For this review, take the finished solid that the model builds, in its own axes (mm). Coordinates: 2 decimals unless noted, no trailing zeros. Write each loop counter-clockwise with the first axis right and the second up, starting at its lowest first coordinate (ties: lowest second). Pieces come first, ordered by that corner, then holes. Notation, with made-up numbers: M -22.5,-39 L 16.5,-39 A33 cw 16.5,-2 Z; hole C -7,-16.75 d3. An arc over 180 degrees is marked long. Return JSON: item names as keys, results as strings.
```python
from build123d import *

# Parameters (mm, degrees)
CYLINDER_R        = 15.5
CYLINDER_DEPTH    = 10
CYLINDER001_R     = 32.5
CYLINDER001_DEPTH = 1


with BuildPart() as cylinder:
    # Cylinder → Cylinder (new body)
    with BuildSketch(Plane.XY.offset(-2)):
        Circle(CYLINDER_R)
    extrude(amount=CYLINDER_DEPTH)


with BuildPart() as cut:
    # Cylinder001 → Cylinder001 (new body)
    with BuildSketch(Plane.XY):
        Circle(CYLINDER001_R)
    extrude(amount=CYLINDER001_DEPTH)

    # Cut: cut Cylinder
    add(cylinder.part, mode=Mode.SUBTRACT)


solid = cut.part
```
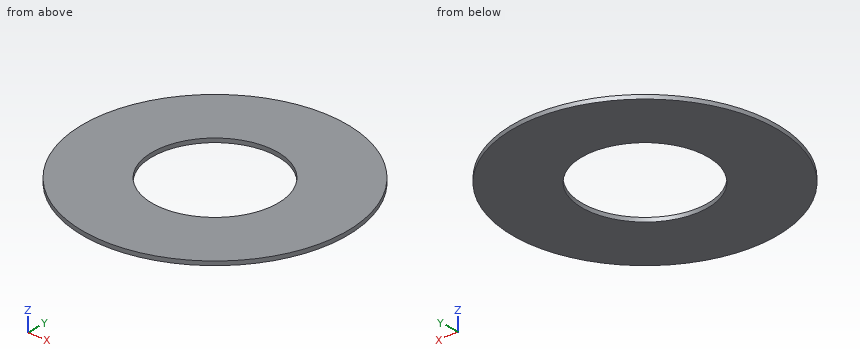
1. We need section D-D (x = -24.5). State the section outline as (y, z) points, plus the area to 3 significant figures.
Checks:
{"outline": "M -21.35,0 L 21.35,0 L 21.35,1 L -21.35,1 Z", "area": "42.7 mm2"}
2. We need section C-C (z = 0.7). State the section outline as (x, y) points, plus the area to 3 significant figures.
Checks:
{"outline": "C 0,0 d65; hole C 0,0 d31", "area": "2,560 mm2"}
3. Wall thickness on L1, parallel to Y at x = 0, z = 0.35; L2, parallel to Y at x = 2.5, z = 0.65; L3, parallel to Y at x = 21.5, z = 0.4: over which ranges is each line inside the solid? List them lowest first. Write a range as from..to.
Checks:
{"L1": "-32.5..-15.5, 15.5..32.5", "L2": "-32.4..-15.3, 15.3..32.4", "L3": "-24.37..24.37"}
4. We need section A-A (x = 0). State the section outline as (y, z) points, plus the area to 3 significant figures.
Checks:
{"outline": "M -32.5,0 L -15.5,0 L -15.5,1 L -32.5,1 Z; M 15.5,0 L 32.5,0 L 32.5,1 L 15.5,1 Z", "area": "34.0 mm2"}
5. Clearance check with a flat-ended pin moving along its axis: pin 1 Ø1.5 at (x, y) = (21, -15) entering from -Z. State where the tip first meets the part, or that it passes through.
Checks:
{"pin 1": "z = 0"}
